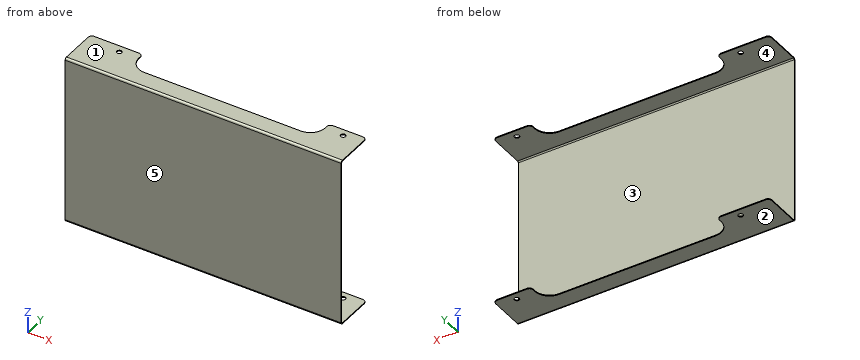
```python
from build123d import *

# Parameters (mm, degrees)
SKETCH_1_W                         = 370
SKETCH_1_H                         = 1.2
SM_BASE_FLANGE_1_DEPTH             = 225
SM_EDGE_FLANGE_1_STRIP_W           = 8
SM_EDGE_FLANGE_1_STRIP_H           = 1.2
SM_EDGE_FLANGE_1_STRIP_CUT_DEPTH   = 370
SM_EDGE_FLANGE_1_STRIP_2_W         = 8
SM_EDGE_FLANGE_1_STRIP_2_H         = 1.2
SM_EDGE_FLANGE_1_STRIP_CUT_2_DEPTH = 370
SM_EDGE_FLANGE_1_DEPTH             = 370
SM_EDGE_FLANGE_1_BEND_DEPTH        = 370
CUT_EXTRUDE_1_DEPTH                = 438.395427502
FILLET_1_R                         = 5
SKETCH_17_R                        = 3.3
CUT_EXTRUDE_2_DEPTH                = 438.395427502


# Sheet-metal steps are written as plain solids
with BuildPart() as part:
    # Sketch 1 → Базовая кромка1 (new body)
    with BuildSketch(Plane.XY):
        with Locations((185, -0.6)):
            Rectangle(SKETCH_1_W, SKETCH_1_H)
    extrude(amount=SM_BASE_FLANGE_1_DEPTH)

    # Ребро-кромка1 strip (across the edge) → Ребро-кромка1 strip cut (cut)
    with BuildSketch(Plane(origin=(0, 0, 225), x_dir=(0, 0, -1), z_dir=(1, 0, 0))):
        with Locations((-2.4, -0.6)):
            Rectangle(SM_EDGE_FLANGE_1_STRIP_W, SM_EDGE_FLANGE_1_STRIP_H)
    extrude(amount=SM_EDGE_FLANGE_1_STRIP_CUT_DEPTH, mode=Mode.SUBTRACT)

    # Ребро-кромка1 strip 2 (across the edge) → Ребро-кромка1 strip cut 2 (cut)
    with BuildSketch(Plane.ZY.offset(-370)):
        with Locations((-2.4, -0.6)):
            Rectangle(SM_EDGE_FLANGE_1_STRIP_2_W, SM_EDGE_FLANGE_1_STRIP_2_H)
    extrude(amount=SM_EDGE_FLANGE_1_STRIP_CUT_2_DEPTH, mode=Mode.SUBTRACT)

    # Ребро-кромка1 section (across the edge) → Ребро-кромка1 (add)
    with BuildSketch(Plane(origin=(0, 0, 225), x_dir=(0, 0, -1), z_dir=(1, 0, 0))):
        with BuildLine():
            Line((-1.2, 1.6), (-1.2, 52))
            Line((-1.2, 52), (0, 52))
            Line((0, 52), (0, 1.6))
            ThreePointArc((0, 1.6), (0.46862915, 0.46862915), (1.6, 0))
            Line((1.6, 0), (1.6, -1.2))
            ThreePointArc((1.6, -1.2), (-0.379898987, -0.379898987), (-1.2, 1.6))
        make_face()
    extrude(amount=SM_EDGE_FLANGE_1_DEPTH)

    # Ребро-кромка1 section 2 (across the edge) → Ребро-кромка1 bend (add)
    with BuildSketch(Plane.ZY.offset(-370)):
        with BuildLine():
            Line((-1.2, 1.6), (-1.2, 52))
            Line((-1.2, 52), (0, 52))
            Line((0, 52), (0, 1.6))
            ThreePointArc((0, 1.6), (0.46862915, 0.46862915), (1.6, 0))
            Line((1.6, 0), (1.6, -1.2))
            ThreePointArc((1.6, -1.2), (-0.379898987, -0.379898987), (-1.2, 1.6))
        make_face()
    extrude(amount=SM_EDGE_FLANGE_1_BEND_DEPTH)

    # Эскиз14 → Вырез-Вытянуть1 (cut, through all)
    with BuildSketch(Plane.XY.offset(226.2)):
        with BuildLine():
            Line((70, 52), (320, 52))
            Line((320, 52), (320, 43.8))
            ThreePointArc((320, 43.8), (314.142135624, 29.657864376), (300, 23.8))
            Line((300, 23.8), (90, 23.8))
            ThreePointArc((90, 23.8), (75.857864376, 29.657864376), (70, 43.8))
            Line((70, 43.8), (70, 52))
        make_face()
    extrude(amount=-CUT_EXTRUDE_1_DEPTH, mode=Mode.SUBTRACT)

    # Скругление1
    fillet_1_edges = [part.edges().sort_by_distance(p)[0] for p in [
        (0, 52, 225.6),
        (370, 52, 225.6),
        (370, 52, -0.6),
        (0, 52, -0.6),
        (70, 52, 225.6),
        (320, 52, 225.6),
        (70, 52, -0.6),
        (320, 52, -0.6),
    ]]
    fillet(fillet_1_edges, radius=FILLET_1_R)

    # Эскиз17 → Вырез-Вытянуть2 (cut, through all)
    with BuildSketch(Plane(origin=(0, 0, -1.2), x_dir=(-1, 0, 0), z_dir=(0, 0, -1))):
        with Locations(Location((-345, 42, 0), (0, 0, 90))):
            Circle(SKETCH_17_R)
        with Locations(Location((-45, 42, 0), (0, 0, 90))):
            Circle(SKETCH_17_R)
    extrude(amount=-CUT_EXTRUDE_2_DEPTH, mode=Mode.SUBTRACT)


solid = part.part
```
Input: part model. Units: mm. Frame: model coordinates. Face numbers are marked on the shaded views. A direction names the side the tool comes from. Give positions to 0.01 mm unless a question says otherwise; leave off trailing zeros. Order: outer loops, then holes, each group sorted by start corner. A loop starts at its lowest first (then second) coordinate and runs counter-clockwise, first axis right, second up. Notation, with made-up numbers: (-18, 65.5) -> (37, 65.5) arc R29 ccw to (37, 97.5) -> close; hole circle Ø7 at (-33.5, -30.75). An arc over 180 degrees is marked (long way). Write each question's results on one line, items separated by ' | '. Start each with the question number.
Item 1: Set-up query: the marked faces 4 and 5. Return all of +Z, -Z, +X, -X, +Y, -Y with unobstructed straight access to the full face (end or side cutting, diameter ignored); none if empty.
Item 2: Line query: line 1 (X direction, y = 42, z = -0.35); line 2 (Z direction, x = 25, y = 24); line 3 (Y direction, x = 315, z = 26). Output: solid intervals per line, ascending.
Item 3: Mould query, pull axis Z, two halves, no side actions, for the marked faces 1, 2 and 3. Classes: pulls with the +Z half, pulls with the -Z half, needs draft (parallel to the pull), parting line crosses it, or undercut.
Item 4: Cut plane D-D on z = 198. Return the cut outline in (x, y), then the cut area to 3 significant figures.
Item 5: Contact query for flat-ended pins moving along their axis: P1, Ø25, axis at x = 120.5, y = 29.5, coming from the +Z side; P2, Ø1.3, axis at x = 201, z = 225.5, coming from the +Y side; P3, Ø2, axis at x = 43, z = 116.5, coming from the +Y side. Output: stop coordinate, or through.
Item 6: Cut plane A-A on x = 34.5. Return the cut outline in (y, z), then the cut area to 3 significant figures.
Item 7: Cut plane B-B on y = 29. Return the cut outline in (x, z), then the cut area to 3 significant figures.
Item 8: Cut plane C-C on x = 147.5. Return the cut outline in (y, z).
Established:
1) face 4: +X, -X, +Y | face 5: +Z, -Z, +X, -X, -Y
2) line 1: 0 to 41.7, 48.3 to 70.08, 319.92 to 341.7, 348.3 to 370 | line 2: -1.2 to 0, 225 to 226.2 | line 3: -1.2 to 0
3) face 1: pulls with the +Z half | face 2: pulls with the -Z half | face 3: undercut
4) outline: (0, -1.2) -> (370, -1.2) -> (370, 0) -> (0, 0) -> close | area: 444 mm^2
5) P1: z = 226.2 | P2: y = 23.8 | P3: y = 0
6) outline: (-1.2, 1.6) arc R2.8 ccw to (1.6, -1.2) -> (52, -1.2) -> (52, 0) -> (1.6, 0) arc R1.6 cw to (0, 1.6) -> (0, 223.4) arc R1.6 cw to (1.6, 225) -> (52, 225) -> (52, 226.2) -> (1.6, 226.2) arc R2.8 ccw to (-1.2, 223.4) -> close | area: 395 mm^2
7) outline: (0, -1.2) -> (76.55, -1.2) -> (76.55, 0) -> (0, 0) -> close; (0, 225) -> (76.55, 225) -> (76.55, 226.2) -> (0, 226.2) -> close; (313.45, -1.2) -> (370, -1.2) -> (370, 0) -> (313.45, 0) -> close; (313.45, 225) -> (370, 225) -> (370, 226.2) -> (313.45, 226.2) -> close | area: 319 mm^2
8) outline: (-1.2, 1.6) arc R2.8 ccw to (1.6, -1.2) -> (23.8, -1.2) -> (23.8, 0) -> (1.6, 0) arc R1.6 cw to (0, 1.6) -> (0, 223.4) arc R1.6 cw to (1.6, 225) -> (23.8, 225) -> (23.8, 226.2) -> (1.6, 226.2) arc R2.8 ccw to (-1.2, 223.4) -> close
